```python
from build123d import *

# Parameters (mm, degrees)
SKETCH1_R           = 2.8575
BOSS_EXTRUDE1_DEPTH = 3.5052
CUT_EXTRUDE1_DEPTH  = 1.9558
SKETCH3_R           = 1.7145
BOSS_EXTRUDE2_DEPTH = 31.75


with BuildPart() as part:
    # Sketch1 → Boss-Extrude1 (new body)
    with BuildSketch(Plane(origin=(0, 0, 0), x_dir=(1, 0, 0), z_dir=(0, 1, 0))):
        Circle(SKETCH1_R)
    extrude(amount=BOSS_EXTRUDE1_DEPTH)

    # Sketch2 → Cut-Extrude1 (cut)
    with BuildSketch(Plane.XZ):
        Polygon((1.603951217, 0), (0.801975608, 1.3890625), (-0.801975608, 1.3890625), (-1.603951217, 0), (-0.801975608, -1.3890625), (0.801975608, -1.3890625), align=None)
    extrude(amount=-CUT_EXTRUDE1_DEPTH, mode=Mode.SUBTRACT)

    # Sketch3 → Boss-Extrude2 (add)
    with BuildSketch(Plane(origin=(0, 3.5052, 0), x_dir=(1, 0, 0), z_dir=(0, 1, 0))):
        Circle(SKETCH3_R)
    extrude(amount=BOSS_EXTRUDE2_DEPTH)


solid = part.part
```
For this review, take the finished solid that the model builds, in its own axes (mm). A direction names the side the tool comes from. Round coordinates to 2 decimals unless told otherwise and drop trailing zeros. Write each loop counter-clockwise with the first axis right and the second up, starting at its lowest first coordinate (ties: lowest second). Pieces come first, ordered by that corner, then holes. Notation, with made-up numbers: (-20, 57) - (16, 57) arc R10 ccw to (16, 61) - close; hole circle Ø9 at (-27.5, 32.25). An arc over 180 degrees is marked (long way). Answer as CSV lines item,"result". Start each with the question number.
(1) Machinability: for faces 1 (the cylindrical face through (2.726, 1.728, -0.858)), 2 (the flat face through (0, 1, -1.389)), 3 (the flat face through (0, 3.505, 2)), which of the approach directions +Z, -Z, +X, -X, +Y, -Y give a long, thin tool a straight path to every point of the face, cutting with its end or side? Answer none if there is none.
(2) Add section D-D, the plane x = -2.3. State the section outline as (y, z) points.
(3) For pin 1 (1 mm diameter, centred on x = -0.5, z = -1.5, fed in from -Y); pin 2 (2 mm diameter, centred on y = 12, z = 0, fed in from -X); pin 3 (1 mm diameter, centred on x = 0.5, y = 30, fed in from +Z), all flat-tipped, find the tip position at first contact; note any pin that passes through.
(4) Add section B-B, the plane y = 4. State the section outline as (x, z) points.
(5) Add section A-A, the plane x = 0. State the section outline as (y, z) points.
(6) Add section C-C, the plane z = -2.25. State the section outline as (x, y) points, plus the area to 3 significant figures.
(7) For line 1 (X direction, y = 22.5, z = -0.1); line 2 (Y direction, x = -0.8, z = -2.25), list the stretches that pass through material, from the lowest coordinate up.
(8) Mouldability with a two-part tool opening along X and no side actions: class faces 4 (the flat face through (0, 35.255, 0)), 5 (the cylindrical face through (-0.372, 19.158, 1.674)), 6 (the flat face through (1.2, 1, -0.7)) as +X half, -X half, draft (parallel to the pull), parting line (faces both ways), or undercut.
From the geometry:
1,face 1,"+Y, -Y"
1,face 2,"-Y"
1,face 3,"+Y"
2,outline,"(0, -1.7) - (3.51, -1.7) - (3.51, 1.7) - (0, 1.7) - close"
3,pin 1,"stops at y = 0"
3,pin 2,"stops at x = -1.71"
3,pin 3,"stops at z = 1.71"
4,outline,"circle Ø3.43 at (0, 0)"
5,outline,"(0, -2.86) - (3.51, -2.86) - (3.51, -1.71) - (35.26, -1.71) - (35.26, 1.71) - (3.51, 1.71) - (3.51, 2.86) - (0, 2.86) - (0, 1.39) - (1.96, 1.39) - (1.96, -1.39) - (0, -1.39) - close"
6,outline,"(-1.76, 0) - (1.76, 0) - (1.76, 3.51) - (-1.76, 3.51) - close"
6,area,"12.3 mm²"
7,line 1,"x = -1.71 to 1.71"
7,line 2,"y = 0 to 3.51"
8,face 4,"draft"
8,face 5,"parting line"
8,face 6,"undercut"
